from build123d import *

# Parameters (mm, degrees)
RESSALTO_EXTRUS_O1_DEPTH = 0.55


with BuildPart() as part:
    # Esboço1 → Ressalto-extrusão1 (new body)
    with BuildSketch(Plane.XY):
        with BuildLine():
            Line((-0.319177055, 12.471030264), (-0.019177055, 12.471030264))
            ThreePointArc((-0.019177055, 12.471030264), (0.051533624, 12.500319586), (0.080822945, 12.571030264))
            Line((0.080822945, 12.571030264), (0.080822945, 14.179397147))
            ThreePointArc((0.080822945, 14.179397147), (0.159639744, 14.382074209), (0.354676223, 14.478255556))
            Line((0.354676223, 14.478255556), (8.354366094, 14.9))
            Line((8.354366094, 14.9), (13.35, 14.9))
            Line((13.35, 14.9), (13.35, 14.7))
            Line((13.35, 14.7), (8.354366094, 14.7))
            Line((8.354366094, 14.7), (0.432418849, 14.285057155))
            Line((0.432418849, 14.285057155), (0.372107371, 14.279016616))
            ThreePointArc((0.372107371, 14.279016616), (0.307095212, 14.246956167), (0.280822945, 14.179397147))
            Line((0.280822945, 14.179397147), (0.280822945, 12.571030264))
            ThreePointArc((0.280822945, 12.571030264), (0.19295498, 12.35889823), (-0.019177055, 12.271030264))
            Line((-0.019177055, 12.271030264), (-0.319177055, 12.271030264))
            Line((-0.319177055, 12.271030264), (-0.319177055, 12.471030264))
        make_face()
    extrude(amount=RESSALTO_EXTRUS_O1_DEPTH)


solid = part.part
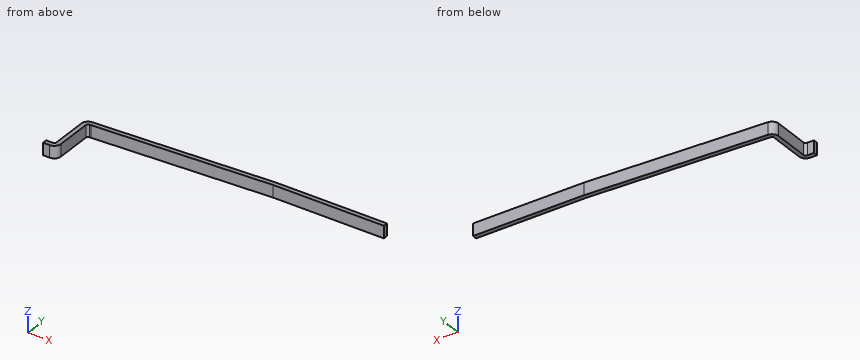
The listing builds one solid part. Answer for the finished solid, in the listing's coordinates (mm). Round coordinates to 2 decimals unless told otherwise and drop trailing zeros. Write each loop counter-clockwise with the first axis right and the second up, starting at its lowest first coordinate (ties: lowest second). Pieces come first, ordered by that corner, then holes. Notation, with made-up numbers: M 62.5,88 L 114.5,88 A22 cw 114.5,121 Z; hole C 5.5,51 d4. An arc over 180 degrees is marked long. Write each question's results on one line, items separated by ' | '. Start each with the question number.
Item 1: Find section A-A on z = 0.1. Write down the section's boundary in (x, y).
Item 2: Find section B-B on x = 9.75. Write down the section's boundary in (y, z), and give its area (3 significant figures).
Item 3: Find section C-C on y = 12.85. Write down the section's boundary in (x, z).
Item 4: Straight lines are drawn through the part: probe 1 along Y at (x, z) = (12.5, 0.2); probe 2 along X at (y, z) = (14, 0.5); probe 3 along Y at (x, z) = (0.5, 0.35). For each, find the intervals that lie inside material, in ascending order.
Answer block:
1) outline: M -0.32,12.27 L -0.02,12.27 A0.3 ccw 0.28,12.57 L 0.28,14.18 A0.1 cw 0.37,14.28 L 0.43,14.29 L 8.35,14.7 L 13.35,14.7 L 13.35,14.9 L 8.35,14.9 L 0.35,14.48 A0.3 ccw 0.08,14.18 L 0.08,12.57 A0.1 cw -0.02,12.47 L -0.32,12.47 Z
2) outline: M 14.7,0 L 14.9,0 L 14.9,0.55 L 14.7,0.55 Z | area: 0.110 mm²
3) outline: M 0.08,0 L 0.28,0 L 0.28,0.55 L 0.08,0.55 Z
4) probe 1: y = 14.7 to 14.9 | probe 2: x = 0.08 to 0.28 | probe 3: y = 14.29 to 14.49
